```python
from build123d import *

# Parameters (mm, degrees)
F0_R     = 9.5
F0_R_2   = 7.5
F1_DEPTH = 3
F0_R_3   = 4.9
F2_DEPTH = 5
F3_DEPTH = 11.5


with BuildPart() as f1:
    # F0 (on Top) → F1 (new body)
    with BuildSketch(Plane.XY):
        Circle(F0_R)
        Circle(F0_R_2, mode=Mode.SUBTRACT)
    extrude(amount=F1_DEPTH)

    # F0 (on Top) → F2 (join)
    with BuildSketch(Plane.XY):
        Circle(F0_R_2)
        Circle(F0_R_3, mode=Mode.SUBTRACT)
    extrude(amount=F2_DEPTH)

    # F0 (on Top) → F3 (join)
    with BuildSketch(Plane.XY):
        Circle(F0_R_3)
        with BuildLine():
            ThreePointArc((-2.2847319318, -2.45), (-3.35, 0), (-2.2847319318, 2.45))
            Line((-2.2847319318, 2.45), (2.2847319318, 2.45))
            ThreePointArc((2.2847319318, 2.45), (3.35, 0), (2.2847319318, -2.45))
            Line((2.2847319318, -2.45), (-2.2847319318, -2.45))
        make_face(mode=Mode.SUBTRACT)
    extrude(amount=F3_DEPTH)

    # F4 (on Front) → F5 (revolve)
    with BuildSketch(Plane.XZ):
        Polygon((5.15, 10.75), (4.9, 11.5), (4.9, 10), align=None)
    revolve(axis=Axis((0, 0, 8.9765712619), (0, 0, 1)))


solid = f1.part
```
Build history of the part. All positions in model axes, mm. A direction names the side the tool comes from. Give positions to 0.01 mm unless a question says otherwise; leave off trailing zeros. Loops run counter-clockwise (first coordinate to the right, second up) from the corner with the lowest first, then second, coordinate; pieces in that order, holes last.
1) Band-saw the part on A-A on y = 0. List the corners of the cut face in (x, z).
Values follow:
outline: (-9.5, 0) - (-3.35, 0) - (-3.35, 11.5) - (-4.9, 11.5) - (-5.15, 10.75) - (-4.9, 10) - (-4.9, 5) - (-7.5, 5) - (-7.5, 3) - (-9.5, 3) - close; (3.35, 0) - (9.5, 0) - (9.5, 3) - (7.5, 3) - (7.5, 5) - (4.9, 5) - (4.9, 10) - (5.15, 10.75) - (4.9, 11.5) - (3.35, 11.5) - close
2) 3-axis set-ups, long thin cutter, end or side, ignore diameter. For faces 4 (the face through (0, -2.45, 6)), 5 (the face through (-7.493, 0.33, 3.986)), 6 (the face through (4, 0, 0)): which of +Z, -Z, +X, -X, +Y, -Y reach the whole face in a straight line?
Values follow:
face 4: +Z, -Z
face 5: +Z
face 6: -Z, +X, -X, +Y, -Y
3) Band-saw the part on C-C on z = 7. List the corners of the cut face in (x, y).
Values follow:
outline: circle Ø9.8 at (0, 0); hole (-2.28, -2.45) - (2.28, -2.45) arc R3.35 ccw to (2.28, 2.45) - (-2.28, 2.45) arc R3.35 ccw to start
4) Band-saw the part on B-B on x = 0. List the corners of the cut face in (y, z).
Values follow:
outline: (-9.5, 0) - (-2.45, 0) - (-2.45, 11.5) - (-4.9, 11.5) - (-5.15, 10.75) - (-4.9, 10) - (-4.9, 5) - (-7.5, 5) - (-7.5, 3) - (-9.5, 3) - close; (2.45, 0) - (9.5, 0) - (9.5, 3) - (7.5, 3) - (7.5, 5) - (4.9, 5) - (4.9, 10) - (5.15, 10.75) - (4.9, 11.5) - (2.45, 11.5) - close
5) Drop flat-ended pins along their axis: P1, Ø3.5, axis at x = -0.5, z = 8, coming from the -Y side; P2, Ø5, axis at x = 1, z = 9, coming from the -Y side; P3, Ø3.5, axis at x = 0, z = 6.5, coming from the +Y side. Give the stop position or say it passes through.
Values follow:
P1: stops at y = -4.9
P2: stops at y = -5.15
P3: stops at y = 7.5
6) Band-saw the part on D-D on y = -5.5. List the corners of the cut face in (x, z), then the cut area to 3 significant figures.
Values follow:
outline: (-7.75, 0) - (7.75, 0) - (7.75, 3) - (5.1, 3) - (5.1, 5) - (-5.1, 5) - (-5.1, 3) - (-7.75, 3) - close
area: 66.9 mm2
7) Probe line 1 along Y through (x, z) = (0.25, 7.75); line 2 along Z through (x, y) = (1, 7.25); line 3 along X through (y, z) = (1.25, 2.5). List the from-to ranges inside material, lowest first.
Values follow:
line 1: y = -4.89 to -2.45, 2.45 to 4.89
line 2: z = 0 to 5
line 3: x = -9.42 to -3.11, 3.11 to 9.42
8) Two-plate mould, pull along Z, no slides. Class faces 1 (the face through (0, -3, 11.5)), 2 (the face through (-1.062, -4.783, 7.465)), 3 (the face through (-3.35, -0.04, 5.67)): released by +Z, released by -Z, zero draft, split by the parting line, or undercut.
Values follow:
face 1: released by +Z
face 2: undercut
face 3: zero draft
